The listing builds one solid part. Answer for the finished solid, in the listing's coordinates (mm). Face numbers are marked on the shaded views. A direction names the side the tool comes from. Give positions to 0.01 mm unless a question says otherwise; leave off trailing zeros. Loops run counter-clockwise (first coordinate to the right, second up) from the corner with the lowest first, then second, coordinate; pieces in that order, holes last. Notation, with made-up numbers: (-34.5, 11.25) - (-16.5, 11.25) arc R28 ccw to (-16.5, 50.25) - close; hole circle Ø11 at (71, 1). An arc over 180 degrees is marked (long way). Answer in a Markdown table with one row per item. Add a question column.
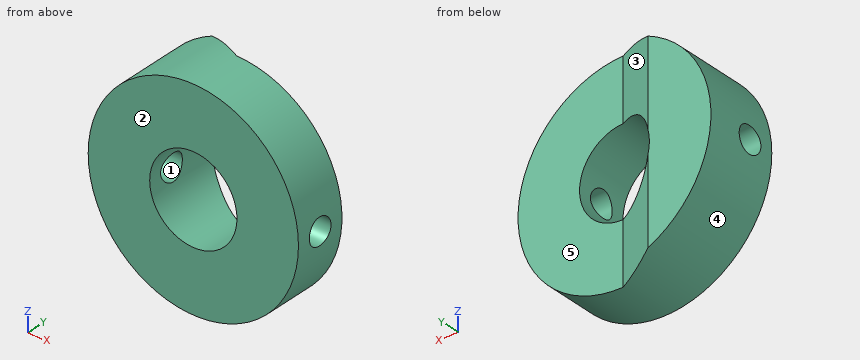
Autodesk Inventor part; units mm, degrees
ref_plane "YZ Plane" through (0, 0, 0) normal (1, 0, 0) x (0, 1, 0)
ref_plane "XZ Plane" through (0, 0, 0) normal (0, 1, 0) x (-1, 0, 0)
ref_plane "XY Plane" through (0, 0, 0) normal (0, 0, 1) x (1, 0, 0)
sketch "Sketch1" plane through (0, 0, 0) normal (0, 1, 0) x (-1, 0, 0)
  circle A0 centre (0, 0) radius 10
  circle A1 centre (0, 0) radius 4.15
  dimension "d0" = 20
  dimension "d1" = 8.3
extrude "Extrusion1" add sketch "Sketch1" along normal blind 5
sketch "Sketch2" plane through (0, 5, 0) normal (0, 1, 0) x (1, 0, 0)
  circle A0 centre (0, 0) radius 4.15 construction
  circle A1 centre (0, 0) radius 10 construction
  circle A2 centre (0, 0) radius 4.15
  line L0 (0, -4.15) -> (0, -10)
  circle A3 centre (0, 0) radius 10
  line L1 (0, 4.15) -> (0, 10)
  line L2 (14, 0) -> (-14, 0) construction
  arc A4 (0, 4.15) -> (0, -4.15) centre (0, 0) ccw construction
  arc A5 (0, 10) -> (0, -10) centre (0, 0) ccw
  arc A6 (0, 4.15) -> (0, -4.15) centre (0, 0) ccw
  line L3 (0, 0) -> (0, -10) construction
  point P0 (0, 4.15)
  dimension "d4" = 90
extrude "Extrusion2" add sketch "Sketch2" along normal blind 2 contours A2 L0 A3 L1 picked at (-0.7977, -7.9531)
chamfer "Chamfer4" distance 4 distance2 2 1 edges at (0, 7, 7.075) measured on face at (-4.6768, 7, -6.482)
chamfer "Chamfer5" distance 4 distance2 2 1 edges at (0, 7, -7.075) measured on face at (-4.7092, 7, 6.0583)
sketch "Sketch3" plane through (0, 0, 0) normal (1, 0, 0) x (0, 1, 0)
  line L0 (5, 4.15) -> (5, -4.15) construction
  line L1 (5, -10) -> (5, 10) construction
  line L2 (0, -10) -> (0, 10) construction
  line L3 (-1.4, 0) -> (8.4, 0) construction
  circle A0 centre (2.5, 0) radius 1.25
  point P0 (0, 0)
  dimension "d22" = 2.5
  dimension "d23" = 2.5
extrude "Extrusion3" cut sketch "Sketch3" along normal through all both and the other way through all
properties part number "ang_wedge"
(1) A cutting plane is placed at C-C on y = 2.5. Determine the outline of the cut face in (x, z).
(2) The mould has two halves that part along Y. Classify the marked faces 1, 2 and 3: pulls with the +Y half, pulls with the -Y half, needs draft (parallel to the pull), parting line crosses it, or undercut.
(3) A cutting plane is placed at B-B on x = 0.25. Determine the outline of the cut face in (y, z).
(4) Find the intervals of material crossed by line 1 along X through (y, z) = (4.5, 0); line 2 along Y through (x, z) = (4, -7); line 3 along Z through (x, y) = (-7.25, 2.5), in increasing order. Write a range as [from, to].
(5) A cutting plane is placed at D-D on x = 5.25. Determine the outline of the cut face in (y, z).
(6) A cutting plane is placed at A-A on z = -2.25. Determine the outline of the cut face in (x, y).
(7) Given pin 1 Ø8 at (x, z) = (3.5, -3) entering from +Y; pin 2 Ø1 at (x, y) = (-1, 5.5) entering from +Z; pin 3 Ø1.5 at (x, z) = (-2.5, 6.5) entering from +Y, each flat-ended and moving along its own axis, determine where each tip first touches the part or whether it passes through.
(8) A tool of negligible diameter and unlimited length cuts with its end or side. For the marked faces 4 and 5, from which of +Z, -Z, +X, -X, +Y, -Y can it reach the whole face along a straight path? Write none if from no direction.
Evaluation:
| question | item | result |
|---|---|---|
| 1 | outline | (-9.92, -1.25) arc R10 ccw to (9.92, -1.25) - (3.96, -1.25) arc R4.15 cw to (-3.96, -1.25) - close; (-9.92, 1.25) - (-3.96, 1.25) arc R4.15 cw to (3.96, 1.25) - (9.92, 1.25) arc R10 ccw to start |
| 2 | face 1 | undercut |
| 2 | face 2 | pulls with the -Y half |
| 2 | face 3 | pulls with the +Y half |
| 3 | outline | (0, -10) - (5, -10) - (5, -4.14) - (0, -4.14) - close; (0, 4.14) - (5, 4.14) - (5, 10) - (0, 10) - close |
| 4 | line 1 | x = [-10, -4.15], [4.15, 10] |
| 4 | line 2 | y = [0, 5] |
| 4 | line 3 | z = [-6.89, -1.25], [1.25, 6.89] |
| 5 | outline | (0, -8.51) - (5, -8.51) - (5, 8.51) - (0, 8.51) - close; hole circle Ø2.5 at (2.5, 0) |
| 6 | outline | (-9.74, 0) - (-3.49, 0) - (-3.49, 6.74) - (-4, 7) - (-9.74, 7) - close; (3.49, 0) - (9.74, 0) - (9.74, 5) - (3.49, 5) - close |
| 7 | pin 1 | stops at y = 5.17 |
| 7 | pin 2 | stops at z = 9.98 |
| 7 | pin 3 | stops at y = 6.63 |
| 8 | face 4 | +Y, -Y |
| 8 | face 5 | +Z, -Z, +X, +Y |
